Design review of the part built by this model. Coordinates are the model's own, in mm. A direction names the side the tool comes from. Give positions to 0.01 mm unless a question says otherwise; leave off trailing zeros. Loops run counter-clockwise (first coordinate to the right, second up) from the corner with the lowest first, then second, coordinate; pieces in that order, holes last. Notation, with made-up numbers: (23, -19.5) -> (46, -19.5) arc R27 cw to (46, 3.5) -> close; hole circle Ø6 at (24.5, -17.75). An arc over 180 degrees is marked (long way). Use CSV: the item, a comma, the result in double quotes. Start each with the question number.
Item 1: We need section C-C (y = 13). State the section outline as (x, z) points, plus the area to 3 significant figures.
Item 2: Clearance check with flat-ended pins moving along their axes: pin 1 (4 mm diameter, centred on y = 0, z = 6.35, fed in from +X); pin 2 (6 mm diameter, centred on y = 14.5, z = -14, fed in from +X); pin 3 (3 mm diameter, centred on x = 11.5, z = -2, fed in from -Y). State where each tip first meets the part, or that it passes through.
Item 3: We need section B-B (x = 3.5). State the section outline as (y, z) points (3 decimals), plus the area to 3 significant figures.
Item 4: We need section D-D (z = 15.5). State the section outline as (x, y) points, plus the area to 3 significant figures.
Item 5: For faces 1 (the face through (0, 8.2, -4)), 2 (the face through (18.62, -0.41, -1.86)), 3 (the face through (7.51, 1.93, -8.68)), list the 3-axis set-ups (+Z, -Z, +X, -X, +Y, -Y) from which the entire face can be reached by the end or side of a thin tool; tool diameter is ignored.
Item 6: Wall thickness on line 1 along Z through (x, y) = (4.5, 7); line 2 along Z through (x, y) = (4, 4); line 3 along Y through (x, z) = (11, -8): over which ranges is each line inside the solid? List them lowest first. Write a range as from..to.
Item 7: The part is to be moulded in two halves that separate along Y. For faces 4 (the face through (21.844, 0, 0)), 5 (the face through (7.51, -15.12, -11.59)), 6 (the face through (0.254, -9, 4)), say which applies: +Y half, -Y half, draft (parallel to the pull), parting line (faces both ways), or undercut.
Item 8: We need section A-A (z = 0). Count the separate pieces of the cut face and the enclosed holes in it, plus the area to 3 significant figures.
from build123d import *

# Parameters (mm, degrees)
F0_R      = 19.05
F1_DEPTH  = 15.24
F2_R      = 18.653125
F3_DEPTH  = 14.986
F4_R      = 9.525
F5_DEPTH  = 15.24
F7_R      = 1.5875
F8_DEPTH  = 2.54
F9_R      = 8.89
F10_DEPTH = 15.24
F11_R     = 1.905
F12_DEPTH = 6.35


# Not quite as in the source:
# - a feature names something its author has since deleted; it is built from what else it names


with BuildPart() as f1:
    # F0 (on Right) → F1 (new body)
    with BuildSketch(Plane.YZ):
        Circle(F0_R)
    extrude(amount=F1_DEPTH)

    # F2 (on face) → F3 (cut)
    with BuildSketch(Plane.YZ.offset(15.24)):
        Circle(F2_R)
    extrude(amount=-F3_DEPTH, mode=Mode.SUBTRACT)

    # F4 (on face) → F5 (join)
    with BuildSketch(Plane.YZ.offset(0.254)):
        Circle(F4_R)
    extrude(amount=F5_DEPTH)

    # F7 (on face) → F8 (cut)
    with BuildSketch(Plane.YZ.offset(15.494)):
        with BuildLine():
            ThreePointArc((1.5875, 6.35), (-1.1225320151, 7.4725320151), (0, 4.7625))
            ThreePointArc((0, 4.7625), (1.1225320151, 5.2274679849), (1.5875, 6.35))
        make_face()
        with BuildLine():
            ThreePointArc((7.9375, 0), (6.35, 1.5875), (4.7625, 0))
            ThreePointArc((4.7625, 0), (6.35, -1.5875), (7.9375, 0))
        make_face()
        with BuildLine():
            ThreePointArc((1.5875, -6.35), (1.1225320151, -5.2274679849), (0, -4.7625))
            ThreePointArc((0, -4.7625), (-1.1225320151, -7.4725320151), (1.5875, -6.35))
        make_face()
        with Locations((-6.35, 0)):
            Circle(F7_R)
        with BuildLine():
            ThreePointArc((6.0059587639, 4.2942080269), (3.8214214188, 5.7651610032), (3.2800341547, 3.187796865))
            ThreePointArc((3.2800341547, 3.187796865), (5.015496109, 2.8232550506), (6.0059587639, 4.2942080269))
        make_face()
        with BuildLine():
            ThreePointArc((6.0059587639, -4.5463046331), (5.0364104329, -3.0840146534), (3.312047602, -3.4078800239))
            ThreePointArc((3.312047602, -3.4078800239), (3.8005070949, -6.0085946128), (6.0059587639, -4.5463046331))
        make_face()
        with BuildLine():
            ThreePointArc((-3.0903496579, -4.5463046331), (-3.2068966816, -3.949267288), (-3.5394250487, -3.4398934712))
            ThreePointArc((-3.5394250487, -3.4398934712), (-6.1488026342, -5.1433419782), (-3.0903496579, -4.5463046331))
        make_face()
        with BuildLine():
            ThreePointArc((-3.0903496579, 4.2942080269), (-6.157153182, 4.8702439055), (-3.5083872434, 3.2206560202))
            ThreePointArc((-3.5083872434, 3.2206560202), (-3.1985461338, 3.7181721482), (-3.0903496579, 4.2942080269))
        make_face()
    extrude(amount=-F8_DEPTH, mode=Mode.SUBTRACT)

    # F9 (on face) → F10 (cut)
    with BuildSketch(Plane(origin=(0, 0, 0), x_dir=(0, -1, 0), z_dir=(-1, 0, 0))):
        Circle(F9_R)
    extrude(amount=-F10_DEPTH, mode=Mode.SUBTRACT)

    # F11 (on face) → F12 (join)
    with BuildSketch(Plane.YZ.offset(15.494)):
        Circle(F11_R)
    extrude(amount=F12_DEPTH)


solid = f1.part
Results found:
1,outline,"(0, -13.92) -> (15.24, -13.92) -> (15.24, -13.38) -> (0.25, -13.38) -> (0.25, 13.38) -> (15.24, 13.38) -> (15.24, 13.92) -> (0, 13.92) -> close"
1,area,"23.5 mm²"
2,pin 1,"x = 15.49"
2,pin 2,"x = 15.24"
2,pin 3,"y = -19.04"
3,outline,"circle Ø38.1 at (0, 0); circle Ø19.05 at (0, 0); hole circle Ø37.306 at (0, 0); hole circle Ø17.78 at (0, 0)"
3,area,"83.7 mm²"
4,outline,"(0, -11.07) -> (15.24, -11.07) -> (15.24, -10.38) -> (0.25, -10.38) -> (0.25, 10.38) -> (15.24, 10.38) -> (15.24, 11.07) -> (0, 11.07) -> close"
4,area,"26.5 mm²"
5,face 1,"+Z, -Z, -X, +Y, -Y"
5,face 2,"+X"
5,face 3,"-X"
6,line 1,"-17.72..-17.29, -6.46..-5.48, 5.48..6.46, 17.29..17.72"
6,line 2,"-18.63..-18.22, -8.64..-7.94, 7.94..8.64, 18.22..18.63"
6,line 3,"-17.29..-16.85, -5.17..-3.88, 3.88..5.17, 16.85..17.29"
7,face 4,"draft"
7,face 5,"parting line"
7,face 6,"undercut"
8,separate pieces,"3"
8,enclosed holes,"0"
8,area,"63.5 mm²"
